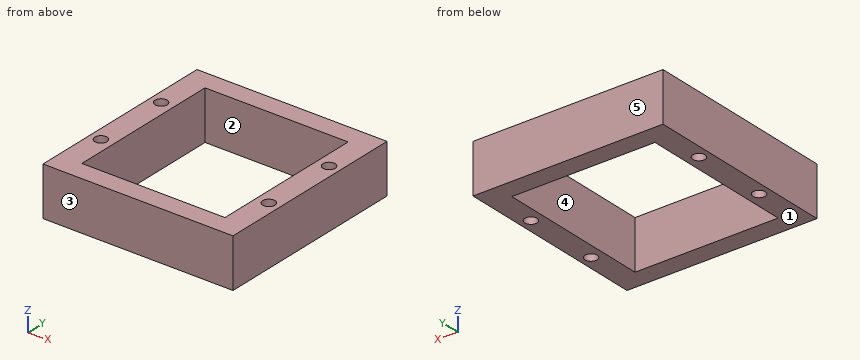
from build123d import *

# Parameters (mm, degrees)
SKETCH1_W           = 31
SKETCH1_H           = 32
BOSS_EXTRUDE1_DEPTH = 8
SKETCH2_W           = 23.35
SKETCH2_H           = 25.6
CUT_EXTRUDE1_DEPTH  = 13
SKETCH3_R           = 1
CUT_EXTRUDE2_DEPTH  = 10


with BuildPart() as part:
    # Sketch1 → Boss-Extrude1 (new body)
    with BuildSketch(Plane.XY):
        Rectangle(SKETCH1_W, SKETCH1_H)
    extrude(amount=BOSS_EXTRUDE1_DEPTH)

    # Sketch2 → Cut-Extrude1 (cut)
    with BuildSketch(Plane.XY.offset(8)):
        Rectangle(SKETCH2_W, SKETCH2_H)
    extrude(amount=-CUT_EXTRUDE1_DEPTH, mode=Mode.SUBTRACT)

    # Sketch3 → Cut-Extrude2 (cut)
    with BuildSketch(Plane.XY.offset(8)):
        with Locations((13.7, 6.25)):
            Circle(SKETCH3_R)
        with Locations((13.7, -6.25)):
            Circle(SKETCH3_R)
        with Locations((-13.7, -6.25)):
            Circle(SKETCH3_R)
        with Locations((-13.7, 6.25)):
            Circle(SKETCH3_R)
    extrude(amount=-CUT_EXTRUDE2_DEPTH, mode=Mode.SUBTRACT)


solid = part.part
For this review, take the finished solid that the model builds, in its own axes (mm). Face numbers are marked on the shaded views. A direction names the side the tool comes from. Round coordinates to 2 decimals unless told otherwise and drop trailing zeros. Write each loop counter-clockwise with the first axis right and the second up, starting at its lowest first coordinate (ties: lowest second). Pieces come first, ordered by that corner, then holes. Notation, with made-up numbers: (44, 21) - (94, 21) arc R15 cw to (94, 49) - close; hole circle Ø7 at (86, 61.25). An arc over 180 degrees is marked (long way). Write item = value, one per line. Start each with the question number.
1. Draft analysis for pull direction Y (two halves, no side actions). For the marked faces 1, 2 and 3, state which applies: released by +Y, released by -Y, zero draft, split by the parting line, or undercut.
2. For the marked faces 4 and 5, list the 3-axis set-ups (+Z, -Z, +X, -X, +Y, -Y) from which the entire face can be reached by the end or side of a thin tool; tool diameter is ignored.
3. Consider section C-C on y = 8. State the section outline as (x, z) points (3 decimals), plus the area to 3 significant figures.
4. Consider section B-B on y = -6.25. State the section outline as (x, z) points (3 decimals).
5. Consider section D-D on z = 5. State the section outline as (x, y) points (3 decimals).
6. Wall thickness on L1, parallel to Y at x = -13.7, z = 4.75; L2, parallel to Y at x = 11.5, z = 3; L3, parallel to X at y = 6.5, z = 6.75 (3 decimals): over which ranges is each line inside the solid? List them lowest first.
7. Consider section A-A on x = -8. State the section outline as (y, z) points, plus the area to 3 significant figures.
Evaluation:
q1.face_1 = zero draft
q1.face_2 = undercut
q1.face_3 = released by -Y
q2.face_4 = +Z, -Z
q2.face_5 = +Z, -Z, +X, -X, +Y
q3.outline = (-15.5, 0) - (-11.675, 0) - (-11.675, 8) - (-15.5, 8) - close; (11.675, 0) - (15.5, 0) - (15.5, 8) - (11.675, 8) - close
q3.area = 61.2 mm2
q4.outline = (-15.5, 0) - (-14.7, 0) - (-14.7, 8) - (-15.5, 8) - close; (-12.7, 0) - (-11.675, 0) - (-11.675, 8) - (-12.7, 8) - close; (11.675, 0) - (12.7, 0) - (12.7, 8) - (11.675, 8) - close; (14.7, 0) - (15.5, 0) - (15.5, 8) - (14.7, 8) - close
q5.outline = (-15.5, -16) - (15.5, -16) - (15.5, 16) - (-15.5, 16) - close; hole circle Ø2 at (-13.7, -6.25); hole circle Ø2 at (-13.7, 6.25); hole (-11.675, -12.8) - (11.675, -12.8) - (11.675, 12.8) - (-11.675, 12.8) - close; hole circle Ø2 at (13.7, -6.25); hole circle Ø2 at (13.7, 6.25)
q6.L1 = -16 to -7.25, -5.25 to 5.25, 7.25 to 16
q6.L2 = -16 to -12.8, 12.8 to 16
q6.L3 = -15.5 to -14.668, -12.732 to -11.675, 11.675 to 12.732, 14.668 to 15.5
q7.outline = (-16, 0) - (-12.8, 0) - (-12.8, 8) - (-16, 8) - close; (12.8, 0) - (16, 0) - (16, 8) - (12.8, 8) - close
q7.area = 51.2 mm2
